```python
from build123d import *

# Parameters (mm, degrees)
SKETCH_1_W           = 70
SKETCH_1_H           = 30
EXTRUDE_1_DEPTH      = 27
CUT_EXTRUDE_1_DEPTH  = 47.679760068
SKETCH_3_R           = 1.65
CUT_EXTRUDE_2_DEPTH  = 47.679760068
SKETCH_4_W           = 21
SKETCH_4_H           = 8.5
CUT_EXTRUDE_3_DEPTH  = 47.679760068
SKETCH_7_R           = 11.25
CUT_EXTRUDE_5_DEPTH  = 47.679760068
SKETCH_8_W           = 21.5
SKETCH_8_H           = 21.5
EXTRUDE_2_DEPTH      = 8
SKETCH_10_R          = 1.5
CUT_EXTRUDE_6_DEPTH  = 54.422841557
SKETCH_12_W          = 35
SKETCH_12_H          = 21.5
EXTRUDE_3_DEPTH      = 3
SKETCH_13_R          = 3
CUT_EXTRUDE_7_DEPTH  = 15
SKETCH_14_R          = 1.65
EXTRUDE_4_DEPTH      = 27
SKETCH_15_W          = 27
SKETCH_15_H          = 30
EXTRUDE_5_DEPTH      = 3
EXTRUDE_START        = 5.5
SKETCH_16_R          = 3
EXTRUDE_6_DEPTH      = 5.5
SKETCH_22_W          = 26
SKETCH_22_H          = 15
CUT_EXTRUDE_9_DEPTH  = 8
EXTRUDE_START_2      = 8
SKETCH_20_R          = 11.25
EXTRUDE_8_DEPTH      = 8
CUT_EXTRUDE_8_DEPTH  = 8
SKETCH_23_W          = 26
SKETCH_23_H          = 20
EXTRUDE_9_DEPTH      = 17
SKETCH_24_R          = 2
CUT_EXTRUDE_10_DEPTH = 64.837684795
SKETCH_25_R          = 3.75
CUT_EXTRUDE_11_DEPTH = 5
SKETCH_26_R          = 3.1
CUT_EXTRUDE_12_DEPTH = 16
SKETCH_27_R          = 1.25
CUT_EXTRUDE_13_DEPTH = 10
SKETCH_28_W          = 2
SKETCH_28_H          = 12.06571985
CUT_EXTRUDE_14_DEPTH = 16
FILLET_1_R           = 2
SKETCH_29_W          = 20
SKETCH_29_H          = 5
CUT_EXTRUDE_15_DEPTH = 89.945207853
SKETCH_30_W          = 8
SKETCH_30_H          = 47.5
CUT_EXTRUDE_16_DEPTH = 87.955448363
SKETCH_31_W          = 15
SKETCH_31_H          = 35.5
CUT_EXTRUDE_17_DEPTH = 87.955448363


with BuildPart() as part:
    # 草图1 → 凸台-拉伸1 (new body)
    with BuildSketch(Plane.XY):
        Rectangle(SKETCH_1_W, SKETCH_1_H)
    extrude(amount=EXTRUDE_1_DEPTH)

    # 草图2 → 切除-拉伸1 (cut, through all)
    with BuildSketch(Plane.XY.offset(27)):
        with BuildLine():
            Line((28.228756555, -15), (35, -15))
            Line((35, -15), (35, 0))
            ThreePointArc((35, 0), (33.228756555, -8.228756555), (28.228756555, -15))
        make_face()
        with BuildLine():
            ThreePointArc((28.228756555, 15), (33.228756555, 8.228756555), (35, 0))
            Line((35, 0), (35, 15))
            Line((35, 15), (28.228756555, 15))
        make_face()
    extrude(amount=-CUT_EXTRUDE_1_DEPTH, mode=Mode.SUBTRACT)

    # 草图3 → 切除-拉伸2 (cut, through all)
    with BuildSketch(Plane.XY.offset(27)):
        with Locations((31, 0)):
            Circle(SKETCH_3_R)
        with Locations((26.313708499, 11.313708499)):
            Circle(SKETCH_3_R)
        with Locations(Location((26.313708499, -11.313708499, 0), (0, 0, 180))):
            Circle(SKETCH_3_R)
        with Locations(Location((3.686291501, 11.313708499, 0), (0, 0, 180))):
            Circle(SKETCH_3_R)
        with Locations((3.686291501, -11.313708499)):
            Circle(SKETCH_3_R)
        with Locations((-1, 0)):
            Circle(SKETCH_3_R)
    extrude(amount=-CUT_EXTRUDE_2_DEPTH, mode=Mode.SUBTRACT)

    # 草图4 → 切除-拉伸3 (cut, through all)
    with BuildSketch(Plane.XY.offset(27)):
        with Locations((-24.5, 10.75)):
            Rectangle(SKETCH_4_W, SKETCH_4_H)
    extrude(amount=-CUT_EXTRUDE_3_DEPTH, mode=Mode.SUBTRACT)

    # 草图7 → 切除-拉伸5 (cut, through all)
    with BuildSketch(Plane(origin=(0, 0, 0), x_dir=(-1, 0, 0), z_dir=(0, 0, -1))):
        with Locations((-15, 0)):
            Circle(SKETCH_7_R)
    extrude(amount=-CUT_EXTRUDE_5_DEPTH, mode=Mode.SUBTRACT)

    # 草图8 → 凸台-拉伸2 (add)
    with BuildSketch(Plane(origin=(0, 0, 0), x_dir=(-1, 0, 0), z_dir=(0, 0, -1))):
        with Locations((24.25, -4.25)):
            Rectangle(SKETCH_8_W, SKETCH_8_H)
    extrude(amount=EXTRUDE_2_DEPTH)

    # 草图10 → 切除-拉伸6 (cut, through all)
    with BuildSketch(Plane.XZ.offset(15)):
        with Locations(Location((-17.5, 19.95, 0), (0, 0, 270))):
            Circle(SKETCH_10_R)
        with Locations(Location((-32.5, 19.95, 0), (0, 0, 270))):
            Circle(SKETCH_10_R)
    extrude(amount=-CUT_EXTRUDE_6_DEPTH, mode=Mode.SUBTRACT)

    # 草图12 → 凸台-拉伸3 (add)
    with BuildSketch(Plane.ZY.offset(35)):
        with Locations((9.5, -4.25)):
            Rectangle(SKETCH_12_W, SKETCH_12_H)
    extrude(amount=EXTRUDE_3_DEPTH)

    # 草图13 → 切除-拉伸7 (cut)
    with BuildSketch(Plane.XZ.offset(15)):
        with Locations(Location((-32.5, 19.95, 0), (0, 0, 270))):
            Circle(SKETCH_13_R)
        with Locations(Location((-17.5, 19.95, 0), (0, 0, 270))):
            Circle(SKETCH_13_R)
    extrude(amount=-CUT_EXTRUDE_7_DEPTH, mode=Mode.SUBTRACT)

    # 草图14 → 凸台-拉伸4 (add)
    with BuildSketch(Plane.XY.offset(27)):
        Polygon((28.228756555, -15), (35, -15), (35, 0), (35, 15), (28.228756555, 15), (28.228756555, 12.920752662), (28.228756555, 9.706664336), (28.228756555, 0), (28.228756555, -9.706664336), (28.228756555, -12.920752662), align=None)
        with Locations((31, 0)):
            Circle(SKETCH_14_R, mode=Mode.SUBTRACT)
    extrude(amount=-EXTRUDE_4_DEPTH)

    # 草图15 → 凸台-拉伸5 (add)
    with BuildSketch(Plane(origin=(35, 0, 0), x_dir=(0, 0, -1), z_dir=(1, 0, 0))):
        with Locations((-13.5, 0)):
            Rectangle(SKETCH_15_W, SKETCH_15_H)
    extrude(amount=EXTRUDE_5_DEPTH)

    # 草图16 → 凸台-拉伸6 (add)
    with BuildSketch(Plane.XZ.offset(15).offset(EXTRUDE_START)):
        Polygon((-13.5, 0), (38, 0), (38, 27), (-38, 27), (-38, -8), (-13.5, -8), align=None)
        with Locations(Location((-32.5, 19.95, 0), (0, 0, 270))):
            Circle(SKETCH_16_R, mode=Mode.SUBTRACT)
        with Locations(Location((-17.5, 19.95, 0), (0, 0, 270))):
            Circle(SKETCH_16_R, mode=Mode.SUBTRACT)
    extrude(amount=-EXTRUDE_6_DEPTH)

    # 草图22 → 切除-拉伸9 (cut)
    with BuildSketch(Plane.XZ.offset(20.5)):
        with Locations((-25, 19.5)):
            Rectangle(SKETCH_22_W, SKETCH_22_H)
    extrude(amount=-CUT_EXTRUDE_9_DEPTH, mode=Mode.SUBTRACT)

    # 草图20 → 凸台-拉伸8 (add)
    with BuildSketch(Plane(origin=(0, 0, 0), x_dir=(-1, 0, 0), z_dir=(0, 0, -1)).offset(EXTRUDE_START_2)):
        Polygon((14, 15), (-38, 15), (-38, -20.5), (13.5, -20.5), (13.5, 6.5), (14, 6.5), align=None)
        with Locations((-15, 0)):
            Circle(SKETCH_20_R, mode=Mode.SUBTRACT)
    extrude(amount=-EXTRUDE_8_DEPTH)

    # 草图21 → 切除-拉伸8 (cut)
    with BuildSketch(Plane(origin=(0, 0, -8), x_dir=(-1, 0, 0), z_dir=(0, 0, -1))):
        with BuildLine():
            Line((-27.816005618, -16), (-2.183994382, -16))
            ThreePointArc((-2.183994382, -16), (-15, 20.5), (-27.816005618, -16))
        make_face()
    extrude(amount=-CUT_EXTRUDE_8_DEPTH, mode=Mode.SUBTRACT)

    # 草图23 → 凸台-拉伸9 (add)
    with BuildSketch(Plane.XZ.offset(20.5)):
        with Locations((-25, 2)):
            Rectangle(SKETCH_23_W, SKETCH_23_H)
    extrude(amount=EXTRUDE_9_DEPTH)

    # 草图24 → 切除-拉伸10 (cut, through all)
    with BuildSketch(Plane(origin=(0, 0, -8), x_dir=(-1, 0, 0), z_dir=(0, 0, -1))):
        with Locations((17, -27)):
            Circle(SKETCH_24_R)
        with Locations((25, -27)):
            Circle(SKETCH_24_R)
    extrude(amount=-CUT_EXTRUDE_10_DEPTH, mode=Mode.SUBTRACT)

    # 草图25 → 切除-拉伸11 (cut)
    with BuildSketch(Plane(origin=(0, 0, -8), x_dir=(-1, 0, 0), z_dir=(0, 0, -1))):
        with Locations((17, -27)):
            Circle(SKETCH_25_R)
        with Locations((25, -27)):
            Circle(SKETCH_25_R)
    extrude(amount=-CUT_EXTRUDE_11_DEPTH, mode=Mode.SUBTRACT)

    # 草图26 → 切除-拉伸12 (cut)
    with BuildSketch(Plane.XZ.offset(37.5)):
        with Locations(Location((-31, 7, 0), (0, 0, 270))):
            Circle(SKETCH_26_R)
    extrude(amount=-CUT_EXTRUDE_12_DEPTH, mode=Mode.SUBTRACT)

    # 草图27 → 切除-拉伸13 (cut)
    with BuildSketch(Plane.XZ.offset(21.5)):
        with Locations(Location((-31, 7, 0), (0, 0, 270))):
            Circle(SKETCH_27_R)
    extrude(amount=-CUT_EXTRUDE_13_DEPTH, mode=Mode.SUBTRACT)

    # 草图28 → 切除-拉伸14 (cut)
    with BuildSketch(Plane.XZ.offset(37.5)):
        with Locations((-31, -1.967140075)):
            Rectangle(SKETCH_28_W, SKETCH_28_H)
    extrude(amount=-CUT_EXTRUDE_14_DEPTH, mode=Mode.SUBTRACT)

    # 圆角1
    fillet_1_edges = [part.edges().sort_by_distance(p)[0] for p in [
        (-32, -29.5, 4.06571985),
        (-30, -29.5, 4.06571985),
    ]]
    fillet(fillet_1_edges, radius=FILLET_1_R)

    # 草图29 → 切除-拉伸15 (cut, through all)
    with BuildSketch(Plane.ZY.offset(38)):
        with Locations((2, -35)):
            Rectangle(SKETCH_29_W, SKETCH_29_H)
    extrude(amount=-CUT_EXTRUDE_15_DEPTH, mode=Mode.SUBTRACT)

    # 草图30 → 切除-拉伸16 (cut, through all)
    with BuildSketch(Plane(origin=(38, 0, 0), x_dir=(0, 0, -1), z_dir=(1, 0, 0))):
        with Locations((4, -8.75)):
            Rectangle(SKETCH_30_W, SKETCH_30_H)
    extrude(amount=-CUT_EXTRUDE_16_DEPTH, mode=Mode.SUBTRACT)

    # 草图31 → 切除-拉伸17 (cut, through all)
    with BuildSketch(Plane.ZY.offset(38)):
        with Locations((19.5, -2.75)):
            Rectangle(SKETCH_31_W, SKETCH_31_H)
    extrude(amount=-CUT_EXTRUDE_17_DEPTH, mode=Mode.SUBTRACT)


solid = part.part
```
For this review, take the finished solid that the model builds, in its own axes (mm). A direction names the side the tool comes from. Round coordinates to 2 decimals unless told otherwise and drop trailing zeros. Write each loop counter-clockwise with the first axis right and the second up, starting at its lowest first coordinate (ties: lowest second). Pieces come first, ordered by that corner, then holes. Notation, with made-up numbers: (82, 9) - (124, 9) arc R19 ccw to (124, 46) - close; hole circle Ø9 at (-34, 34). An arc over 180 degrees is marked (long way). Answer as a JSON object with one key per item and string values.
1. To check wall thickness, follow line 1 along X through (y, z) = (-24.5, 7.25); line 2 along X through (y, z) = (1.5, 2); line 3 along X through (y, z) = (-21, 7). State the ranges of each line that lie inside material, in increasing order.
Response values:
{"line 1": "x = -38 to -34.09, -27.91 to -12", "line 2": "x = -38 to -1.69, -0.31 to 3.85, 26.15 to 30.31, 31.69 to 38", "line 3": "x = -38 to -32.25, -29.75 to -12"}
2. Draft analysis for pull direction Z (two halves, no side actions). For faces 6 (the face through (-32.22, -26.92, 3.79)), 7 (the face through (27.838, 10.682, 6.084)), 8 (the face through (1, -9, 0)), state which applies: +Z half, -Z half, draft (parallel to the pull), parting line (faces both ways), or undercut.
Response values:
{"face 6": "undercut", "face 7": "draft", "face 8": "-Z half"}
3. We need section C-C on z = 7. Count the separate pieces of the cut face and the enclosed holes in it, then the cut area to 3 significant figures.
Response values:
{"separate pieces": "1", "enclosed holes": "9", "area": "2,240 mm2"}
4. We need section B-B on y = -27. Give the boundary of the cut face in (x, z).
Response values:
{"outline": "(-38, 0) - (-32, 0) - (-32, 2.88) arc R2 ccw to (-32.82, 4.49) arc R3.1 cw (long way) to (-29.18, 4.49) arc R2 ccw to (-30, 2.88) - (-30, 0) - (-27, 0) - (-27, 12) - (-38, 12) - close; (-23, 0) - (-19, 0) - (-19, 12) - (-23, 12) - close; (-15, 0) - (-12, 0) - (-12, 12) - (-15, 12) - close"}
5. We need section D-D on y = -2.5. Give the boundary of the cut face in (x, z).
Response values:
{"outline": "(-38, 0) - (4.03, 0) - (4.03, 12) - (-38, 12) - close; (25.97, 0) - (38, 0) - (38, 12) - (25.97, 12) - close"}
6. Tool access review of faces 1 (the face through (-12, -26, 6)), 2 (the face through (-30, -27, 1)), 3 (the face through (4.4, -12.8, 6.1)), 4 (the face through (-30.155, -16.57, 7.921)), 5 (the face through (-14, 11, 6)): name each direction out of +Z, -Z, +X, -X, +Y, -Y from which nothing blocks a thin tool from reaching the whole face with its end or side.
Response values:
{"face 1": "+Z, -Z, +X, -Y", "face 2": "-Z, -Y", "face 3": "+Z, -Z", "face 4": "-Y", "face 5": "+Z, -Z, -X, +Y"}
7. For pin 1 Ø6 at (x, z) = (15, 6.5) entering from -Y; pin 2 Ø0.9 at (y, z) = (-26.5, 1.5) entering from +X; pin 3 Ø2.5 at (y, z) = (13, 5.5) entering from -X, all flat-tipped, find the tip position at first contact; note any pin that passes through.
Response values:
{"pin 1": "stops at y = -20.5", "pin 2": "stops at x = -12", "pin 3": "stops at x = -14"}
8. We need section A-A on x = -25. Give the boundary of the cut face in (y, z), then the cut area to 3 significant figures.
Response values:
{"outline": "(-32.5, 0) - (-29, 0) - (-29, 12) - (-32.5, 12) - close; (-25, 0) - (6.5, 0) - (6.5, 12) - (-25, 12) - close", "area": "420 mm2"}
